from build123d import *

# Parameters (mm, degrees)
EXTRUDE_1_DEPTH     = 25
SKETCH_2_R          = 1.5
CUT_EXTRUDE_1_DEPTH = 52.203275929
SKETCH_3_R          = 5
CUT_EXTRUDE_2_DEPTH = 48.891361585


with BuildPart() as part:
    # 草图1 → 凸台-拉伸1 (new body)
    with BuildSketch(Plane.XY):
        Polygon((-11.527836019, 18.697603401), (-11.527836019, -19.302396599), (26.472163981, -19.302396599), (26.472163981, -17.302396599), (-9.527836019, -17.302396599), (-9.527836019, 18.697603401), align=None)
    extrude(amount=EXTRUDE_1_DEPTH)

    # 草图2 → 切除-拉伸1 (cut, through all)
    with BuildSketch(Plane(origin=(0, -17.302396599, 0), x_dir=(1, 0, 0), z_dir=(0, 1, 0))):
        with Locations(Location((-1.527836019, -5, 0), (0, 0, 180))):
            Circle(SKETCH_2_R)
        with Locations(Location((8.472163981, -5, 0), (0, 0, 180))):
            Circle(SKETCH_2_R)
        with Locations(Location((8.472163981, -20, 0), (0, 0, 180))):
            Circle(SKETCH_2_R)
        with Locations(Location((-1.527836019, -20, 0), (0, 0, 180))):
            Circle(SKETCH_2_R)
    extrude(amount=-CUT_EXTRUDE_1_DEPTH, mode=Mode.SUBTRACT)

    # 草图3 → 切除-拉伸2 (cut, through all)
    with BuildSketch(Plane(origin=(-9.527836019, 0, 0), x_dir=(0, 0, -1), z_dir=(1, 0, 0))):
        with Locations(Location((-12.5, -1.302396599, 0), (0, 0, 90))):
            Circle(SKETCH_3_R)
    extrude(amount=-CUT_EXTRUDE_2_DEPTH, mode=Mode.SUBTRACT)


solid = part.part
CAD build for the part. Positions are in the model's coordinates, mm. A direction names the side the tool comes from. Give positions to 0.01 mm unless a question says otherwise; leave off trailing zeros. Write each loop counter-clockwise with the first axis right and the second up, starting at its lowest first coordinate (ties: lowest second). Pieces come first, ordered by that corner, then holes. Notation, with made-up numbers: (-1.75, 80) - (31.25, 80) arc R23 ccw to (31.25, 100) - close; hole circle Ø11 at (3, -8.5). An arc over 180 degrees is marked (long way). Put each result on its own line as item: value.
(1) Pull direction X, two halves, no side cores. Call faces 1 (the flat face through (-11, -9, 25)), 2 (the cylindrical face through (8.667, -18.288, 21.487)), 3 (the flat face through (26.472, -18, 12)): released by +X, released by -X, zero draft, split by the parting line, or undercut.
Working result:
face 1: zero draft
face 2: undercut
face 3: released by +X
(2) Tool access for faces 4 (the cylindrical face through (-0.03, -18.29, 5.07)), 5 (the flat face through (9, -17.302, 12)): list every direction of +Z, -Z, +X, -X, +Y, -Y with a clear straight run to the whole face (end or side of a thin tool).
Working result:
face 4: +Y, -Y
face 5: +Z, -Z, +X, +Y
(3) Saw through at D-D (y = 2). List the corners of the cut face in (x, z), then the cut area to 3 significant figures.
Working result:
outline: (-11.53, 0) - (-9.53, 0) - (-9.53, 8.75) - (-11.53, 8.75) - close; (-11.53, 16.25) - (-9.53, 16.25) - (-9.53, 25) - (-11.53, 25) - close
area: 35.0 mm^2
(4) Drop flat-ended pins along their axis: pin 1 Ø7.5 at (y, z) = (-7, 7.5) entering from +X; pin 2 Ø1.5 at (x, z) = (8, 14) entering from +Y. Give the stop position or say it passes through.
Working result:
pin 1: x = -9.53
pin 2: y = -17.3
(5) Wall check: L1, parallel to X at y = -2, z = 5; L2, parallel to Y at x = 25, z = 20.5. Give the ranges that are in metal, low to high.
Working result:
L1: -11.53 to -9.53
L2: -19.3 to -17.3
(6) Saw through at B-B (z = 5). List the corners of the cut face in (x, y), then the cut area to 3 significant figures.
Working result:
outline: (-11.53, -19.3) - (-3.03, -19.3) - (-3.03, -17.3) - (-9.53, -17.3) - (-9.53, 18.7) - (-11.53, 18.7) - close; (-0.03, -19.3) - (6.97, -19.3) - (6.97, -17.3) - (-0.03, -17.3) - close; (9.97, -19.3) - (26.47, -19.3) - (26.47, -17.3) - (9.97, -17.3) - close
area: 136 mm^2
(7) Saw through at A-A (z = 12.5). List the corners of the cut face in (x, y).
Working result:
outline: (-11.53, -19.3) - (26.47, -19.3) - (26.47, -17.3) - (-9.53, -17.3) - (-9.53, -6.3) - (-11.53, -6.3) - close; (-11.53, 3.7) - (-9.53, 3.7) - (-9.53, 18.7) - (-11.53, 18.7) - close
(8) Saw through at C-C (x = -1.5). List the corners of the cut face in (y, z).
Working result:
outline: (-19.3, 0) - (-17.3, 0) - (-17.3, 3.5) - (-19.3, 3.5) - close; (-19.3, 6.5) - (-17.3, 6.5) - (-17.3, 18.5) - (-19.3, 18.5) - close; (-19.3, 21.5) - (-17.3, 21.5) - (-17.3, 25) - (-19.3, 25) - close
